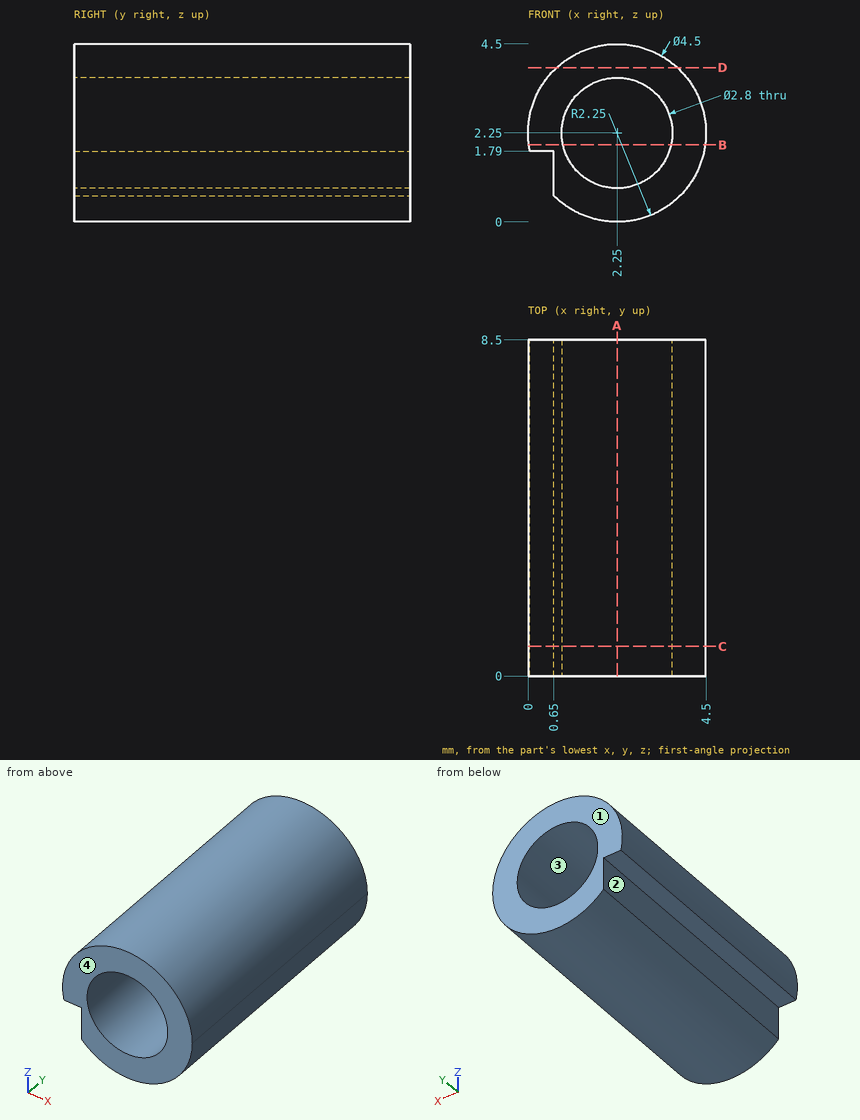
The figure shows three views and two pictorial views of one solid part (mm, origin at its lowest corner). Answer the questions. A direction names the side the tool comes from. Give positions to 0.01 mm unless a question says otherwise; leave off trailing zeros. Loops run counter-clockwise (first coordinate to the right, second up) from the corner with the lowest first, then second, coordinate; pieces in that order, holes last. Notation, with made-up numbers: (40.25, 51) - (63.25, 51) arc R32 cw to (63.25, 90) - close; hole circle Ø5 at (-18, 87.5). An arc over 180 degrees is marked (long way). Use one line per item in the form item = value.
1. Find the intervals of material crossed by line 1 along Z through (x, y) = (2.25, 2.25); line 2 along X through (y, z) = (2.75, 1.1); line 3 along X through (y, z) = (8, 1.85), in increasing order. Write a range as [from, to].
Calculated:
line_1 = [0, 0.85], [3.65, 4.5]
line_2 = [0.65, 1.45], [3.05, 4.18]
line_3 = [0.04, 0.91], [3.59, 4.46]
2. Which of the six approach directions +Z, -Z, +X, -X, +Y, -Y give full straight-line access (tool end or side, diameter ignored) to the marked faces 1 and 2?
Calculated:
face_1 = +Z, -Z, +X, -X, +Y
face_2 = -Z, -X, +Y, -Y
3. Section A-A on x = 2.25 is taken. Give the vertices of the cut face in (y, z).
Calculated:
outline = (0, 0) - (8.5, 0) - (8.5, 0.85) - (0, 0.85) - close; (0, 3.65) - (8.5, 3.65) - (8.5, 4.5) - (0, 4.5) - close
4. Section C-C on y = 0.75 is taken. Give the vertices of the cut face in (x, z).
Calculated:
outline = (0.05, 1.79) - (0.65, 1.79) - (0.65, 0.67) arc R2.25 ccw (long way) to start; hole circle Ø2.8 at (2.25, 2.25)
5. Section D-D on z = 3.9 is taken. Give the vertices of the cut face in (x, y), then the cut area to 3 significant figures.
Calculated:
outline = (0.72, 0) - (3.78, 0) - (3.78, 8.5) - (0.72, 8.5) - close
area = 26.0 mm^2
6. The mould has two halves that part along Z. Classify the marked faces 3 and 4: pulls with the +Z half, pulls with the -Z half, needs draft (parallel to the pull), parting line crosses it, or undercut.
Calculated:
face_3 = undercut
face_4 = needs draft
7. Section B-B on z = 1.95 is taken. Give the vertices of the cut face in (x, y).
Calculated:
outline = (0.02, 0) - (0.88, 0) - (0.88, 8.5) - (0.02, 8.5) - close; (3.62, 0) - (4.48, 0) - (4.48, 8.5) - (3.62, 8.5) - close
8. Given pin 1 Ø1.5 at (y, z) = (6, 1) entering from +X; pin 2 Ø0.9 at (y, z) = (4, 1.5) entering from -X; pin 3 Ø1.7 at (x, z) = (2.25, 2.25) entering from -Y, each flat-ended and moving along its own axis, determine where each tip first touches the part or whether it passes through.
Calculated:
pin_1 = 4.44
pin_2 = 0.02
pin_3 = through
